Solid Edge part; units mm, degrees
sketch "Sketch1" plane through (0, 0, 0) normal (0, 0, 1) x (1, 0, 0)
  line L0 (-16, -12) -> (16, -12)
  line L1 (16, -12) -> (16, 12)
  line L2 (16, 12) -> (-16, 12)
  line L3 (-16, 12) -> (-16, -12)
  dimension "D1" = 16
  dimension "D2" = 16
extrude "Protrusion1" add sketch "Sketch1" along normal blind 12
sketch "Sketch2" plane through (0, 0, 12) normal (0, 0, 1) x (0, 1, 0)
  line L0 (-6.1, 16) -> (6.1, 16)
  line L1 (6.1, 16) -> (6.1, -10)
  line L2 (6.1, -10) -> (-6.1, -10)
  line L3 (-6.1, -10) -> (-6.1, 16)
  dimension "D1" = 6.1
  dimension "D2" = 6.1
extrude "servo_cutout" cut sketch "Sketch2" against normal blind 6
hole "screw_bearing" at (4, 0, 0) direction (0, 0, 1) diameter 4.7 depth 30 tip angle 118 start chamfer 0.6 start chamfer angle 45 end chamfer 0.6 end chamfer angle 45
chamfer "Chamfer1" distance 0.5 angle 45 5 edges at (-3, -6.1, 12) (-16, -6.1, 9) (10, 0, 12) (-3, 6.1, 12) (-16, 6.1, 9)
hole "Hole1" at (-9.2, 9, 12) direction (0, 0, -1) diameter 2.8 depth 30 tip angle 118 start chamfer 0.3 start chamfer angle 45 end chamfer 0.3 end chamfer angle 45
hole "Hole2" at (-9.2, -9, 12) direction (0, 0, -1) diameter 2.8 depth 30 tip angle 118 start chamfer 0.3 start chamfer angle 45 end chamfer 0.3 end chamfer angle 45
chamfer "Chamfer2" distance 2 angle 45 7 edges at (16, 12, 6) (0, 12, 0) (16, 0, 0) (0, -12, 0) (16, -12, 6) (-16, 12, 6) (-16, -12, 6)
properties material "Polypropylene, general purpose"
Geometry: final body of the model. Coordinates: model frame, mm. A direction names the side the tool comes from. Round coordinates to 2 decimals unless told otherwise and drop trailing zeros. Write each loop counter-clockwise with the first axis right and the second up, starting at its lowest first coordinate (ties: lowest second). Pieces come first, ordered by that corner, then holes.
Item 1: Pin query (flat end, axial travel): P1, Ø1.6, axis at y = 3, z = 8, coming from the -X side. Return the tip coordinate at first contact, or that it passes through.
Item 2: Section query C-C (y = -9). Return loops of the section in (x, z), plus the area to 3 significant figures.
Item 3: Section query B-B (z = 3.5). Return loops of the section in (x, y).
Item 4: Mould query, pull axis X, two halves, no side actions, for faces 3 (the face through (10, 0, 9)), 4 (the face through (-9.14, 7.48, 0.18)), 5 (the face through (0, 8, 12)). Classes: +X half, -X half, draft (parallel to the pull), parting line (faces both ways), or undercut.
Item 5: Material intervals for L1, parallel to Y at x = -9.2, z = 5.5; L2, parallel to Y at x = -9.2, z = 9.25; L3, parallel to X at y = -9, z = 9, sorted ascending.
Item 6: Set-up query: faces 1 (the face through (0, 12, 7)), 2 (the face through (-3, 0, 6)). Return all of +Z, -Z, +X, -X, +Y, -Y with unobstructed straight access to the full face (end or side cutting, diameter ignored); none if empty.
Item 7: Section query D-D (z = 8). Return loops of the section in (x, y).
Item 8: Section query A-A (x = -9.2). Return loops of the section in (y, z), plus the area to 3 significant figures.
Completed:
1. P1: stops at x = 10
2. outline: (-16, 0) - (-10.9, 0) - (-10.6, 0.3) - (-10.6, 11.7) - (-10.9, 12) - (-16, 12) - close; (-7.8, 0.3) - (-7.5, 0) - (14, 0) - (16, 2) - (16, 12) - (-7.5, 12) - (-7.8, 11.7) - close
2. area: 348 mm2
3. outline: (-16, -10) - (-14, -12) - (14, -12) - (16, -10) - (16, 10) - (14, 12) - (-14, 12) - (-16, 10) - close; hole circle Ø2.8 at (-9.2, -9); hole circle Ø2.8 at (-9.2, 9); hole circle Ø4.7 at (4, 0)
4. face 3: -X half
4. face 4: undercut
4. face 5: draft
5. L1: y = -12 to -10.4, -7.6 to 7.6, 10.4 to 12
5. L2: y = -12 to -10.4, -7.6 to -6.1, 6.1 to 7.6, 10.4 to 12
5. L3: x = -16 to -10.6, -7.8 to 16
6. face 1: +Z, -Z, +X, -X, +Y
6. face 2: +Z, -X
7. outline: (-16, -10) - (-14, -12) - (14, -12) - (16, -10) - (16, 10) - (14, 12) - (-14, 12) - (-16, 10) - (-16, 6.6) - (-15.5, 6.1) - (10, 6.1) - (10, -6.1) - (-15.5, -6.1) - (-16, -6.6) - close; hole circle Ø2.8 at (-9.2, -9); hole circle Ø2.8 at (-9.2, 9)
8. outline: (-12, 2) - (-10.4, 0.4) - (-10.4, 11.7) - (-10.7, 12) - (-12, 12) - close; (-7.6, 0.3) - (-7.3, 0) - (7.3, 0) - (7.6, 0.3) - (7.6, 11.7) - (7.3, 12) - (6.6, 12) - (6.1, 11.5) - (6.1, 6) - (-6.1, 6) - (-6.1, 11.5) - (-6.6, 12) - (-7.3, 12) - (-7.6, 11.7) - close; (10.4, 0.4) - (12, 2) - (12, 12) - (10.7, 12) - (10.4, 11.7) - close
8. area: 143 mm2
